```python
from build123d import *

# Parameters (mm, degrees)
F0_W      = 480
F0_H      = 682
F1_DEPTH  = 12
F2_W      = 6
F2_H      = 682
F3_DEPTH  = 6
F4_W      = 474
F4_H      = 6
F5_DEPTH  = 6
F6_W      = 6
F6_H      = 66
F7_DEPTH  = 6
F8_W      = 474
F8_H      = 6
F9_DEPTH  = 6
F10_W     = 400
F10_H     = 130
F11_DEPTH = 12
F12_W     = 474
F12_H     = 6
F13_DEPTH = 6


with BuildPart() as f1:
    # F0 (on Right) → F1 (new body)
    with BuildSketch(Plane.YZ):
        Rectangle(F0_W, F0_H)
    extrude(amount=F1_DEPTH)

    # F2 (on face) → F3 (cut)
    with BuildSketch(Plane(origin=(0, 0, 0), x_dir=(0, -1, 0), z_dir=(-1, 0, 0))):
        with Locations((237, 0)):
            Rectangle(F2_W, F2_H)
    extrude(amount=-F3_DEPTH, mode=Mode.SUBTRACT)

    # F4 (on face) → F5 (cut)
    with BuildSketch(Plane(origin=(0, 0, 0), x_dir=(0, -1, 0), z_dir=(-1, 0, 0))):
        with Locations((-3, 338)):
            Rectangle(F4_W, F4_H)
    extrude(amount=-F5_DEPTH, mode=Mode.SUBTRACT)

    # F6 (on face) → F7 (cut)
    with BuildSketch(Plane(origin=(0, 0, 0), x_dir=(0, -1, 0), z_dir=(-1, 0, 0))):
        with Locations((-237, 302)):
            Rectangle(F6_W, F6_H)
    extrude(amount=-F7_DEPTH, mode=Mode.SUBTRACT)

    # F8 (on face) → F9 (cut)
    with BuildSketch(Plane(origin=(0, 0, 0), x_dir=(0, -1, 0), z_dir=(-1, 0, 0))):
        with Locations((-3, -108)):
            Rectangle(F8_W, F8_H)
    extrude(amount=-F9_DEPTH, mode=Mode.SUBTRACT)

    # F10 (on face) → F11 (cut, through all)
    with BuildSketch(Plane.YZ.offset(12)):
        with Locations((6, -226)):
            Rectangle(F10_W, F10_H)
    extrude(amount=-F11_DEPTH, mode=Mode.SUBTRACT)

    # F12 (on face) → F13 (cut)
    with BuildSketch(Plane(origin=(0, 0, 0), x_dir=(0, -1, 0), z_dir=(-1, 0, 0))):
        with Locations((-3, -338)):
            Rectangle(F12_W, F12_H)
    extrude(amount=-F13_DEPTH, mode=Mode.SUBTRACT)


solid = f1.part
```
The listing builds one solid part. Answer for the finished solid, in the listing's coordinates (mm). Round coordinates to 2 decimals unless told otherwise and drop trailing zeros. Loops run counter-clockwise (first coordinate to the right, second up) from the corner with the lowest first, then second, coordinate; pieces in that order, holes last. Notation, with made-up numbers: (-14, 64) - (1, 64) arc R15 ccw to (1, 81) - close; hole circle Ø7 at (-8.75, 51.5). An arc over 180 degrees is marked (long way). Use one line per item in the form item = value. Start each with the question number.
1. The part is cut by section B-B on z = -263. Determine the outline of the cut face in (x, y), then the cut area to 3 significant figures.
2. Given pin 1 Ø3 at (x, y) = (4, 67) entering from -Z; pin 2 Ø5 at (y, z) = (-82.5, 31) entering from -X; pin 3 Ø1.8 at (x, z) = (1.5, 27) entering from -Y; pin 4 Ø5 at (x, y) = (3, -176.5) entering from +Z, each flat-ended and moving along its own axis, determine where each tip first touches the part or whether it passes through.
3. The part is cut by section A-A on x = 2. Determine the outline of the cut face in (y, z).
4. Consider line 1 (Z direction, x = 5.25, y = -101); line 2 (Y direction, x = 11.5, z = -288); line 3 (Y direction, x = 5, z = -238). Determine where each line is inside the solid, lowest interval first. Write a range as [from, to].
5. The part is cut by section C-C on y = -183. Determine the outline of the cut face in (x, z), then the cut area to 3 significant figures.
Geometry check:
q1.outline = (0, -234) - (6, -234) - (6, -240) - (12, -240) - (12, -194) - (0, -194) - close; (0, 206) - (12, 206) - (12, 240) - (0, 240) - close
q1.area = 924 mm^2
q2.pin_1 = -335
q2.pin_2 = 0
q2.pin_3 = -234
q2.pin_4 = 335
q3.outline = (-234, -335) - (240, -335) - (240, -111) - (-234, -111) - close; (-234, -105) - (240, -105) - (240, 269) - (234, 269) - (234, 335) - (-234, 335) - close; hole (-194, -291) - (206, -291) - (206, -161) - (-194, -161) - close
q4.line_1 = [-335, -291], [-161, -111], [-105, 335]
q4.line_2 = [-240, -194], [206, 240]
q4.line_3 = [-234, -194], [206, 240]
q5.outline = (0, -335) - (6, -335) - (6, -341) - (12, -341) - (12, -291) - (0, -291) - close; (0, -161) - (12, -161) - (12, 341) - (6, 341) - (6, 335) - (0, 335) - (0, -105) - (6, -105) - (6, -111) - (0, -111) - close
q5.area = 6,520 mm^2
